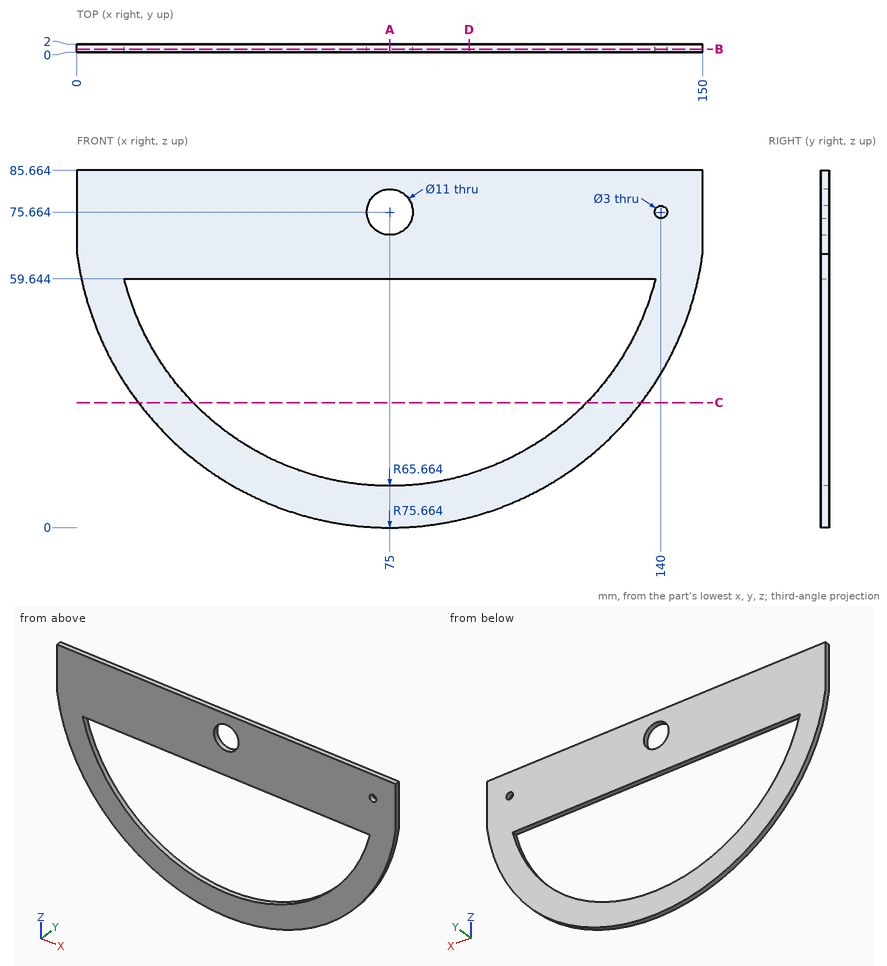
Geometry: see drawing. Coordinates: mm, zero at the bounding-box minimum. Give positions to 0.01 mm unless a question says otherwise; leave off trailing zeros. Order: outer loops, then holes, each group sorted by start corner. A loop starts at its lowest first (then second) coordinate and runs counter-clockwise, first axis right, second up.
1. Cut plane C-C (z = 30). Return loops of the section in (x, y).
Computed:
outline: (14.67, 0) - (27.81, 0) - (27.81, 2) - (14.67, 2) - close; (122.19, 0) - (135.33, 0) - (135.33, 2) - (122.19, 2) - close
2. Cut plane D-D (x = 94). Return loops of the section in (y, z) (1 decimal).
Computed:
outline: (0, 2.4) - (2, 2.4) - (2, 12.8) - (0, 12.8) - close; (0, 59.6) - (2, 59.6) - (2, 85.7) - (0, 85.7) - close
3. Pin query (flat end, axial travel): pin 1 Ø2.5 at (x, z) = (140, 75.66) entering from -Y. Return the tip coordinate at first contact, or that it passes through.
Computed:
pin 1: passes through
4. Line query: probe 1 along X at (y, z) = (0.95, 54.5); probe 2 along Z at (x, y) = (18, 0.8) (1 decimal); probe 3 along X at (y, z) = (0.2, 15) (1 decimal). Output: solid intervals per line, ascending.
Computed:
probe 1: x = 2.36 to 12.84, 137.16 to 147.64
probe 2: z = 25.9 to 43.1, 59.6 to 85.7
probe 3: x = 29.8 to 49.9, 100.1 to 120.2
5. Cut plane A-A (x = 75). Return loops of the section in (y, z) (1 decimal).
Computed:
outline: (0, 0) - (2, 0) - (2, 10) - (0, 10) - close; (0, 59.6) - (2, 59.6) - (2, 70.2) - (0, 70.2) - close; (0, 81.2) - (2, 81.2) - (2, 85.7) - (0, 85.7) - close
6. Cut plane B-B (y = 0.75). Return loops of the section in (x, z) (1 decimal).
Computed:
outline: (0, 65.7) arc R75.7 ccw to (150, 65.7) - (150, 85.7) - (0, 85.7) - close; hole (11.3, 59.6) arc R65.7 ccw to (138.7, 59.6) - close; hole circle Ø11 at (75, 75.7); hole circle Ø3 at (140, 75.7)
